Read the model definition and answer for the solid it produces. Units are mm, in the model's axes. A direction names the side the tool comes from. Give positions to 0.01 mm unless a question says otherwise; leave off trailing zeros. Order: outer loops, then holes, each group sorted by start corner. A loop starts at its lowest first (then second) coordinate and runs counter-clockwise, first axis right, second up. Notation, with made-up numbers: (54, 22) -> (83, 22) arc R17 cw to (83, 49) -> close; hole circle Ø8 at (52.5, -39). An arc over 180 degrees is marked (long way). Use one line per item in the form item = value.
Autodesk Inventor part; units mm, degrees
ref_plane "YZ Plane" through (0, 0, 0) normal (1, 0, 0) x (0, 1, 0)
ref_plane "XZ Plane" through (0, 0, 0) normal (0, 1, 0) x (-1, 0, 0)
ref_plane "XY Plane" through (0, 0, 0) normal (0, 0, 1) x (1, 0, 0)
sketch "スケッチ1" plane through (0, 0, 0) normal (0, 0, 1) x (1, 0, 0)
  circle A0 centre (0, 0) radius 16
  dimension "d0" = 32
extrude "押し出し1" add sketch "スケッチ1" along normal blind 4
sketch "スケッチ2" plane through (0, 0, 4) normal (0, 0, 1) x (1, 0, 0)
  circle A0 centre (0, 0) radius 13.5
  dimension "d3" = 27
extrude "押し出し2" add sketch "スケッチ2" along normal blind 5
sketch "スケッチ3" plane through (0, 0, 9) normal (0, 0, 1) x (1, 0, 0)
  circle A0 centre (0, 0) radius 7.5
  dimension "d6" = 15
extrude "押し出し3" cut sketch "スケッチ3" against normal through all
fillet "フィレット1" radius 0.1 2 edges at (-16, 0, 4) (-16, 0, 0)
properties part number "555_GearBox_Flange" material "鉄、鋳鉄"
Item 1: The part is cut by section D-D on z = 3. Give the vertices of the cut face in (x, y), and give its area (3 significant figures).
Checks:
outline = circle Ø32 at (0, 0); hole circle Ø15 at (0, 0)
area = 628 mm²
Item 2: The part is cut by section C-C on z = 6.75. Give the vertices of the cut face in (x, y), and give its area (3 significant figures).
Checks:
outline = circle Ø27 at (0, 0); hole circle Ø15 at (0, 0)
area = 396 mm²
Item 3: Which of the six approach directions +Z, -Z, +X, -X, +Y, -Y give full straight-line access (tool end or side, diameter ignored) to faces 4 (the flat face through (7, 4, 0)), 5 (the flat face through (-7, -12, 4))?
Checks:
face_4 = -Z, +X, -X, +Y, -Y
face_5 = +Z
Item 4: Straight lines are drawn through the part: L1, parallel to Y at x = 0, z = 6.75; L2, parallel to Z at x = 3.5, y = -13.5; L3, parallel to Y at x = 3.5, z = 1. For each, find the intervals that lie inside material, in ascending order. Write a range as from..to.
Checks:
L1 = -13.5..-7.5, 7.5..13.5
L2 = 0..4
L3 = -15.61..-6.63, 6.63..15.61
Item 5: Given pin 1 Ø5 at (x, z) = (-11.5, 4) entering from -Y; pin 2 Ø12 at (x, y) = (0, 9.5) entering from -Z; pin 3 Ø5 at (y, z) = (-2, 7.5) entering from +X; pin 4 Ø3 at (x, z) = (-8.5, 3) entering from -Y, each flat-ended and moving along its own axis, determine where each tip first touches the part or whether it passes through.
Checks:
pin_1 = -13.23
pin_2 = 0
pin_3 = 13.5
pin_4 = -14.39
Item 6: Determine the mould class of faces 1 (the cylindrical face through (-7.493, 0.33, 4.563)), 2 (the flat face through (6, -6, 9)), 3 (the cylindrical face through (-3.47, 15.62, 1.97)) for opening direction Y: +Y half, -Y half, draft (parallel to the pull), parting line (faces both ways), or undercut.
Checks:
face_1 = undercut
face_2 = draft
face_3 = parting line
Item 7: The part is cut by section A-A on x = 0. Give the vertices of the cut face in (y, z).
Checks:
outline = (-16, 0.1) arc R0.1 ccw to (-15.9, 0) -> (-7.5, 0) -> (-7.5, 9) -> (-13.5, 9) -> (-13.5, 4) -> (-15.9, 4) arc R0.1 ccw to (-16, 3.9) -> close; (7.5, 0) -> (15.9, 0) arc R0.1 ccw to (16, 0.1) -> (16, 3.9) arc R0.1 ccw to (15.9, 4) -> (13.5, 4) -> (13.5, 9) -> (7.5, 9) -> close
